Could you check a few things on this model? Use its own coordinates, in mm. Give positions to 0.01 mm unless a question says otherwise; leave off trailing zeros. Write each loop counter-clockwise with the first axis right and the second up, starting at its lowest first coordinate (ties: lowest second). Pieces come first, ordered by that corner, then holes. Notation, with made-up numbers: (66.25, 62) - (87.25, 62) arc R21 ccw to (87.25, 92) - close; hole circle Ø11 at (-39.5, 39). An arc over 180 degrees is marked (long way). Use one line per item in the form item = value.
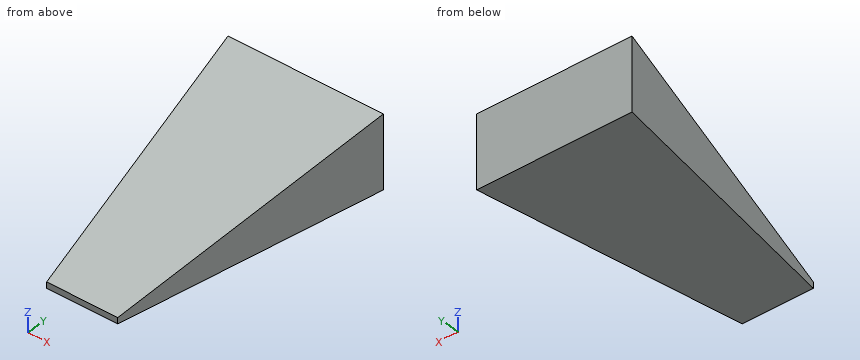
```python
from build123d import *

# Parameters (mm, degrees)
SKETCH_1_W          = 6.5
SKETCH_1_H          = 11
EXTRUDE_1_DEPTH     = 3
CUT_EXTRUDE_1_DEPTH = 10
CUT_EXTRUDE_2_DEPTH = 10


with BuildPart() as part:
    # 草图1 → 凸台-拉伸1 (new body)
    with BuildSketch(Plane.XY):
        with Locations((3.25, -5.5)):
            Rectangle(SKETCH_1_W, SKETCH_1_H)
    extrude(amount=EXTRUDE_1_DEPTH)

    # 草图2 → 切除-拉伸1 (cut)
    with BuildSketch(Plane(origin=(6.5, 0, 0), x_dir=(0, 0, -1), z_dir=(1, 0, 0))):
        Polygon((-3, 0), (-0.252978195, -11), (-3, -11), align=None)
    extrude(amount=-CUT_EXTRUDE_1_DEPTH, mode=Mode.SUBTRACT)

    # 草图3 → 切除-拉伸2 (cut)
    with BuildSketch(Plane(origin=(0, 0, 0), x_dir=(-1, 0, 0), z_dir=(0, 0, -1))):
        Polygon((-6.5, 0), (-4.73741155, -11), (-6.5, -11), align=None)
        Polygon((-1.76258845, -11), (0, -11), (0, 0), align=None)
    extrude(amount=-CUT_EXTRUDE_2_DEPTH, mode=Mode.SUBTRACT)


solid = part.part
```
1. If I drill on line 1 (Z direction, x = 3, y = -3.25); line 2 (Z direction, x = 3.25, y = -5.75); line 3 (X direction, y = -1.25, z = 0.6), over which ranges is the centre line in solid material (lowest first)? Write a range as from..to.
Response values:
line_1 = 0..2.19
line_2 = 0..1.56
line_3 = 0.2..6.3
2. Imagine slicing it at A-A, the plane x = 3.5. List the corners of the cut face in (y, z) for me.
Response values:
outline = (-11, 0) - (0, 0) - (0, 3) - (-11, 0.25) - close
3. Imagine slicing it at B-B, the plane z = 1.4. List the corners of the cut face in (x, y) for me.
Response values:
outline = (0, 0) - (1.03, -6.41) - (5.47, -6.41) - (6.5, 0) - close
4. For pin 1 (1 mm diameter, centred on y = -4, z = 1.5, fed in from +X), with a flat end and sliding along its axis, tell me the tip position at first contact or that it passes through.
Response values:
pin_1 = 5.94
